Here's the drawing with two shaded views (mm, measured from the low corner). I have some questions. Give positions to 0.01 mm unless a question says otherwise; leave off trailing zeros. Order: outer loops, then holes, each group sorted by start corner. A loop starts at its lowest first (then second) coordinate and runs counter-clockwise, first axis right, second up. Notation, with made-up numbers: M -25.75,8 L 25.25,8 A17 cw 25.25,32 Z; hole C 46,11 d11. An arc over 180 degrees is marked long. Use a Markdown table: item, result. Add a question column.
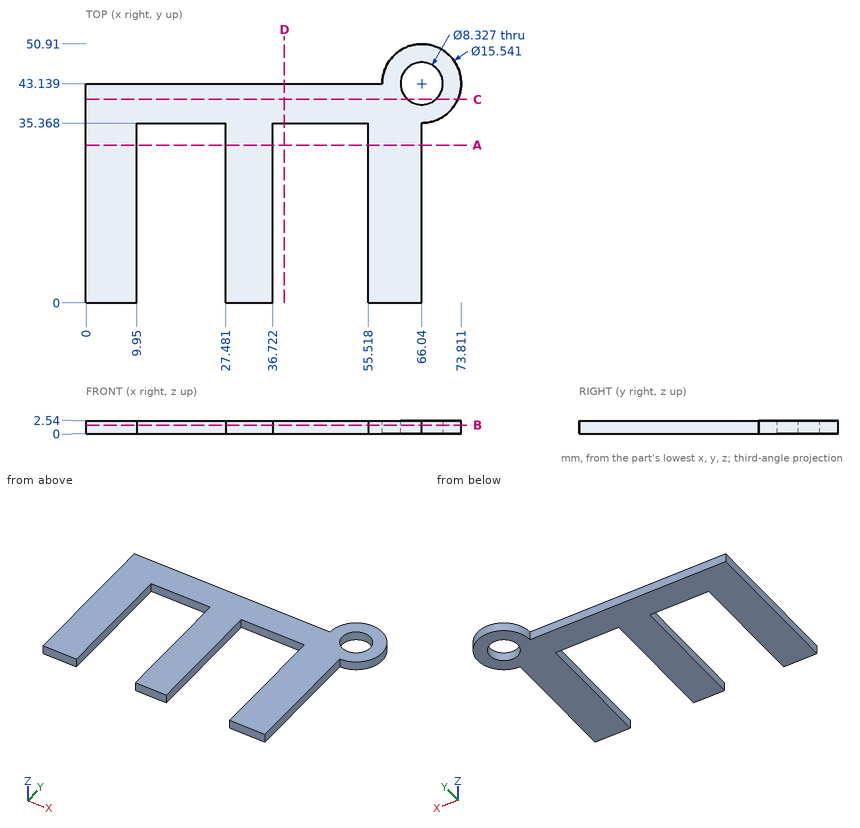
1) Suppose I cut it at D-D on x = 39. Please give me the cut outline in (y, z).
2) Please list where these lines run through material, in increasing order: line 1 (X direction, y = 17, z = 2.3); line 2 (X direction, y = 43, z = 0.1); line 3 (Y direction, x = 50.5, z = 2.05). Write a range as from..to.
3) Suppose I cut it at A-A on y = 31. Please give me the cut outline in (x, z).
4) For pin 1 (1 mm diameter, centred on x = 42, z = 1, fed in from +Y); pin 2 (1.3 mm diameter, centred on y = 25, z = 2, fed in from +X); pin 3 (7.5 mm diameter, centred on x = 66.04, y = 43.14, fed in from +Z); pin 4 (1.3 mm diameter, centred on x = 22, z = 1, fed in from -Y), each with a flat end and sliding along its axis, tell me the tip position at first contact or that it passes through.
5) Suppose I cut it at C-C on y = 40. Please give me the cut outline in (x, z) (1 decimal).
6) Suppose I cut it at B-B on z = 1.7. Please give me the cut outline in (x, y).
Values found:
| question | item | result |
|---|---|---|
| 1 | outline | M 35.37,0 L 43.14,0 L 43.14,2.54 L 35.37,2.54 Z |
| 2 | line 1 | x = 0..9.95, 27.48..36.72, 55.52..66.04 |
| 2 | line 2 | x = 0..61.88, 70.2..73.81 |
| 2 | line 3 | y = 35.37..43.14 |
| 3 | outline | M 0,0 L 9.95,0 L 9.95,2.54 L 0,2.54 Z; M 27.48,0 L 36.72,0 L 36.72,2.54 L 27.48,2.54 Z; M 55.52,0 L 66.04,0 L 66.04,2.54 L 55.52,2.54 Z |
| 4 | pin 1 | stops at y = 43.14 |
| 4 | pin 2 | stops at x = 66.04 |
| 4 | pin 3 | passes through |
| 4 | pin 4 | stops at y = 35.37 |
| 5 | outline | M 0,0 L 63.3,0 L 63.3,2.5 L 0,2.5 Z; M 68.8,0 L 73.1,0 L 73.1,2.5 L 68.8,2.5 Z |
| 6 | outline | M 0,0 L 9.95,0 L 9.95,35.37 L 27.48,35.37 L 27.48,0 L 36.72,0 L 36.72,35.37 L 55.52,35.37 L 55.52,0 L 66.04,0 L 66.04,35.37 A7.77 ccw long 58.27,43.14 L 0,43.14 Z; hole C 66.04,43.14 d8.33 |
